from build123d import *

# Parameters (mm, degrees)
F5_DEPTH = 25


with BuildPart() as f3:
    # F2 (on offset) → F3 section 0
    with BuildSketch(Plane.XY.offset(88)):
        with BuildLine():
            Line((-82.5, 206.5), (-82.5, -206.5))
            ThreePointArc((-82.5, -206.5), (-76.9350288425, -219.9350288425), (-63.5, -225.5))
            Line((-63.5, -225.5), (63.5, -225.5))
            ThreePointArc((63.5, -225.5), (76.9350288425, -219.9350288425), (82.5, -206.5))
            Line((82.5, -206.5), (82.5, 206.5))
            ThreePointArc((82.5, 206.5), (76.9350288425, 219.9350288425), (63.5, 225.5))
            Line((63.5, 225.5), (-63.5, 225.5))
            ThreePointArc((-63.5, 225.5), (-76.9350288425, 219.9350288425), (-82.5, 206.5))
        make_face()
    # F0 (on Top) → F3 section 1
    with BuildSketch(Plane.XY):
        with BuildLine():
            ThreePointArc((78.5, 206.5), (74.1066017178, 217.1066017178), (63.5, 221.5))
            Line((63.5, 221.5), (-63.5, 221.5))
            ThreePointArc((-63.5, 221.5), (-74.1066017178, 217.1066017178), (-78.5, 206.5))
            Line((-78.5, 206.5), (-78.5, -206.5))
            ThreePointArc((-78.5, -206.5), (-74.1066017178, -217.1066017178), (-63.5, -221.5))
            Line((-63.5, -221.5), (63.5, -221.5))
            ThreePointArc((63.5, -221.5), (74.1066017178, -217.1066017178), (78.5, -206.5))
            Line((78.5, -206.5), (78.5, 206.5))
        make_face()
    loft()

    # F4 (on face) → F5 (join)
    with BuildSketch(Plane.XY.offset(88)):
        with BuildLine():
            Line((63.5, 237.5), (-63.5, 237.5))
            ThreePointArc((-63.5, 237.5), (-85.4203102168, 228.4203102168), (-94.5, 206.5))
            Line((-94.5, 206.5), (-94.5, -206.5))
            ThreePointArc((-94.5, -206.5), (-85.4203102168, -228.4203102168), (-63.5, -237.5))
            Line((-63.5, -237.5), (63.5, -237.5))
            ThreePointArc((63.5, -237.5), (85.4203102168, -228.4203102168), (94.5, -206.5))
            Line((94.5, -206.5), (94.5, 206.5))
            ThreePointArc((94.5, 206.5), (85.4203102168, 228.4203102168), (63.5, 237.5))
        make_face()
    extrude(amount=F5_DEPTH)


solid = f3.part
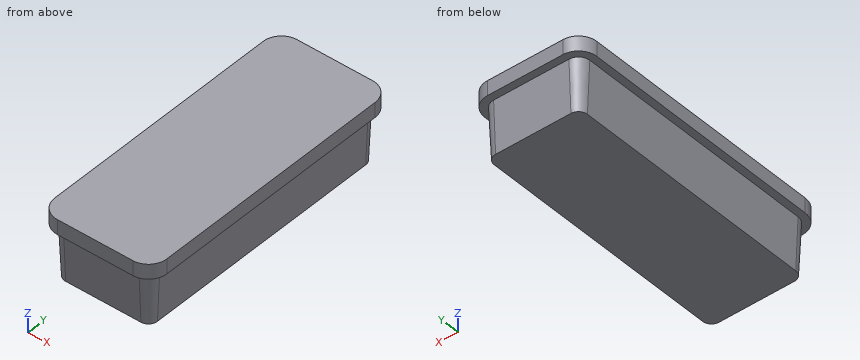
Source: CAD feature listing. Evaluate the final solid. Frame: model axes, mm. Give positions to 0.01 mm unless a question says otherwise; leave off trailing zeros. Write each loop counter-clockwise with the first axis right and the second up, starting at its lowest first coordinate (ties: lowest second). Pieces come first, ordered by that corner, then holes. Notation, with made-up numbers: (-39, -38.5) - (-6, -38.5) arc R23 ccw to (-6, -4.5) - close; hole circle Ø1 at (-7.5, -16.5). An arc over 180 degrees is marked (long way). Write item = value, one per line. Start each with the question number.
Q1. Material intervals for probe 1 along X at (y, z) = (32, 87.5); probe 2 along X at (y, z) = (96, 13); probe 3 along Y at (x, z) = (49.5, 22), sorted ascending.
Q2. Cut plane A-A, the plane x = -38.5. Return loops of the section in (y, z).
Q3. Pin query (flat end, axial travel): pin 1 Ø2 at (x, z) = (62, 54) entering from +Y; pin 2 Ø2 at (x, z) = (-62, 59) entering from +Y; pin 3 Ø6 at (y, z) = (146, 45.5) entering from -X. Return the tip coordinate at first contact, or that it passes through.
Q4. Cut plane B-B, the plane z = 77. Return loops of the section in (x, y).
Computed values:
q1.probe_1 = -82.48 to 82.48
q1.probe_2 = -79.09 to 79.09
q1.probe_3 = -222.5 to 222.5
q2.outline = (-237.5, 88) - (-225.5, 88) - (-221.5, 0) - (221.5, 0) - (225.5, 88) - (237.5, 88) - (237.5, 113) - (-237.5, 113) - close
q3.pin_1 = 224
q3.pin_2 = 224.23
q3.pin_3 = -80.7
q4.outline = (-82, -206.5) arc R18.5 ccw to (-63.5, -225) - (63.5, -225) arc R18.5 ccw to (82, -206.5) - (82, 206.5) arc R18.5 ccw to (63.5, 225) - (-63.5, 225) arc R18.5 ccw to (-82, 206.5) - close
